Geometry check sheet. Reference: the model listing, model coordinates, mm. Face numbers are marked on the shaded views. A direction names the side the tool comes from. Coordinates: 2 decimals unless noted, no trailing zeros. Order: outer loops, then holes, each group sorted by start corner. A loop starts at its lowest first (then second) coordinate and runs counter-clockwise, first axis right, second up. Notation, with made-up numbers: (31, 39) - (50, 39) arc R14 cw to (50, 63) - close; hole circle Ø1 at (-16, 42). An arc over 180 degrees is marked (long way). Use CSV: the item, a comma, the result in double quotes. Start each with the question number.
1) Depth check by flat-ended pin: P1, Ø2.5, axis at x = -3, z = 3.5, coming from the +Y side; P2, Ø6.5, axis at x = -4, y = -2, coming from the -Z side; P3, Ø2.5, axis at y = 10.88, z = 20, coming from the +X side; P4, Ø6, axis at x = 8.5, z = 23, coming from the +Y side. Enter the tip coordinate at first touch or a pass-through.
2) Tool access check on the marked faces 1, 2 and 3. Record the directions out of +Z, -Z, +X, -X, +Y, -Y that give a thin tool (end or side, any length) a straight path to the whole face; none if there is none.
3) Draft check along Z on the marked faces 4, 5 and 6. Enter one of: released by +Z, released by -Z, zero draft, split by the parting line, or undercut.
4) Sectioned sample at C-C, the plane y = 3. Record the cut outline in (x, z), and give its area (3 significant figures).
5) Sectioned sample at B-B, the plane x = 4.25. Record the cut outline in (y, z).
6) Sectioned sample at A-A, the plane z = 36. Record the cut outline in (x, y), and give its area (3 significant figures).
7) Thickness scan on probe 1 along Z at (x, y) = (0, -9.65); probe 2 along Y at (x, z) = (3.6, 20); probe 3 along X at (y, z) = (13, 31). Record the ranges inside material, lowest first. Write a range as [from, to].
8) Sectioned sample at D-D, the plane x = 0. Record the cut outline in (y, z).
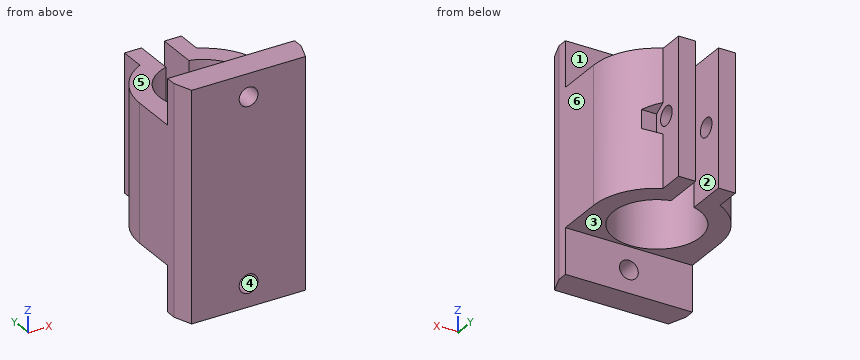
from build123d import *

# Parameters (mm, degrees)
RESSALTO_EXTRUS_O1_DEPTH   = 40
ESBO_O2_W                  = 22.3
ESBO_O2_H                  = 8
CORTE_EXTRUS_O1_DEPTH      = 22.383935
ESBO_O3_R                  = 1.65
CORTE_EXTRUS_O2_DEPTH      = 5
ESBO_O4_R                  = 1.65
CORTE_EXTRUS_O3_DEPTH      = 7.15
CORTE_EXTRUS_O3_DEPTH_BACK = 17.15
ESBO_O5_R                  = 3.5
CORTE_EXTRUS_O4_DEPTH      = 10
CORTE_EXTRUS_O5_DEPTH      = 10
CHANFRO1_SIZE              = 1.15
CHANFRO1_SIZE2             = 3.159599032


with BuildPart() as part:
    # Esboço1 → Ressalto-extrusão1 (new body)
    with BuildSketch(Plane.XY):
        with BuildLine():
            Line((5, 14.383935265), (5, 9.966067429))
            ThreePointArc((5, 9.966067429), (9.488743331, 5.855446183), (11.15, 0))
            Line((11.15, 0), (11.15, -13))
            Line((11.15, -13), (-11.15, -13))
            Line((-11.15, -13), (-11.15, 0))
            ThreePointArc((-11.15, 0), (-9.488743331, 5.855446183), (-5, 9.966067429))
            Line((-5, 9.966067429), (-5, 14.383935265))
            Line((-5, 14.383935265), (-2, 14.383935265))
            Line((-2, 14.383935265), (-2, 7.383935265))
            ThreePointArc((-2, 7.383935265), (0, -7.65), (2, 7.383935265))
            Line((2, 7.383935265), (2, 14.383935265))
            Line((2, 14.383935265), (5, 14.383935265))
        make_face()
    extrude(amount=RESSALTO_EXTRUS_O1_DEPTH)

    # Esboço2 → Corte-extrusão1 (cut)
    with BuildSketch(Plane(origin=(0, 14.383935265, 0), x_dir=(1, 0, 0), z_dir=(0, 1, 0))):
        with Locations((0, -36)):
            Rectangle(ESBO_O2_W, ESBO_O2_H)
        with Locations((0, -4)):
            Rectangle(ESBO_O2_W, ESBO_O2_H)
    extrude(amount=-CORTE_EXTRUS_O1_DEPTH, mode=Mode.SUBTRACT)

    # Esboço3 → Corte-extrusão2 (cut)
    with BuildSketch(Plane(origin=(0, -8, 0), x_dir=(1, 0, 0), z_dir=(0, 1, 0))):
        with Locations((0, -4)):
            Circle(ESBO_O3_R)
        with Locations((0, -36)):
            Circle(ESBO_O3_R)
    extrude(amount=-CORTE_EXTRUS_O2_DEPTH, mode=Mode.SUBTRACT)

    # Esboço4 → Corte-extrusão3 (cut, two sides)
    with BuildSketch(Plane.ZY.offset(5)) as corte_extrus_o3_sk:
        with Locations((20, 10.883935265)):
            Circle(ESBO_O4_R)
    extrude(amount=CORTE_EXTRUS_O3_DEPTH, mode=Mode.SUBTRACT)
    extrude(corte_extrus_o3_sk.sketch, amount=-CORTE_EXTRUS_O3_DEPTH_BACK, mode=Mode.SUBTRACT)

    # Esboço5 → Corte-extrusão4 (cut)
    with BuildSketch(Plane.ZY.offset(5)):
        with Locations((20, 10.883935265)):
            Circle(ESBO_O5_R)
    extrude(amount=CORTE_EXTRUS_O4_DEPTH, mode=Mode.SUBTRACT)

    # Esboço6 → Corte-extrusão5 (cut)
    with BuildSketch(Plane(origin=(5, 0, 0), x_dir=(0, 0, -1), z_dir=(1, 0, 0))):
        Polygon((-16.766838493, 10.883935265), (-18.383419246, 13.683935265), (-21.616580754, 13.683935265), (-23.233161507, 10.883935265), (-21.616580754, 8.083935265), (-18.383419246, 8.083935265), align=None)
    extrude(amount=CORTE_EXTRUS_O5_DEPTH, mode=Mode.SUBTRACT)

    # Chanfro1
    chanfro1_edges = [part.edges().sort_by_distance(p)[0] for p in [
        (11.15, -13, 20),
        (-11.15, -13, 20),
    ]]
    chanfro1_side = [part.faces().sort_by_distance(p)[0] for p in [
        (0, -13, 20),
    ]]
    chamfer(chanfro1_edges, length=CHANFRO1_SIZE, length2=CHANFRO1_SIZE2, reference=chanfro1_side[0])


solid = part.part
Evaluation:
1,P1,"y = -8"
1,P2,"z = 8"
1,P3,"through"
1,P4,"y = 9.7"
2,face 1,"+Z, +X, -X, +Y"
2,face 2,"+Z, -Z, +Y"
2,face 3,"-Z, +X, -X, +Y"
3,face 4,"undercut"
3,face 5,"released by +Z"
3,face 6,"zero draft"
4,outline,"(-10.74, 8) - (-7.04, 8) - (-7.04, 32) - (-10.74, 32) - close; (7.04, 8) - (10.74, 8) - (10.74, 32) - (7.04, 32) - close"
4,area,"178 mm²"
5,outline,"(-13, 0) - (-8, 0) - (-8, 8) - (-6.36, 8) - (-6.36, 32) - (-8, 32) - (-8, 40) - (-13, 40) - close; (6.36, 8) - (14.38, 8) - (14.38, 32) - (6.36, 32) - close; hole circle Ø3.3 at (10.88, 20)"
6,outline,"(-11.15, -9.84) - (-10, -13) - (-1.65, -13) - (-1.65, -8) - (-11.15, -8) - close; (1.65, -13) - (10, -13) - (11.15, -9.84) - (11.15, -8) - (1.65, -8) - close"
6,area,"91.4 mm²"
7,probe 1,"[0, 2.35], [5.65, 34.35], [37.65, 40]"
7,probe 2,"[-13, -6.75], [6.75, 9.23], [12.53, 14.38]"
7,probe 3,"[-5, -2], [2, 5]"
8,outline,"(-13, 0) - (-8, 0) - (-8, 2.35) - (-13, 2.35) - close; (-13, 5.65) - (-8, 5.65) - (-8, 8) - (-7.65, 8) - (-7.65, 32) - (-8, 32) - (-8, 34.35) - (-13, 34.35) - close; (-13, 37.65) - (-8, 37.65) - (-8, 40) - (-13, 40) - close"
